```python
from build123d import *

# Parameters (mm, degrees)
F0_R     = 63.5
F0_R_2   = 44.45
F1_DEPTH = 127
F3_DEPTH = 19.05
F4_W     = 254
F4_H     = 50.8
F5_DEPTH = 152.4
F7_DEPTH = 88.9


with BuildPart() as f1:
    # F0 (on Front) → F1 (new body)
    with BuildSketch(Plane.XZ):
        Circle(F0_R)
        Circle(F0_R_2, mode=Mode.SUBTRACT)
    extrude(amount=F1_DEPTH)

    # F2 (on Front) → F3 (join)
    with BuildSketch(Plane.XZ):
        with BuildLine():
            ThreePointArc((59.227747, 22.898122), (0, -63.5), (-59.227747, 22.898122))
            Line((-59.227747, 22.898122), (-127, -152.4))
            Line((-127, -152.4), (127, -152.4))
            Line((127, -152.4), (59.227747, 22.898122))
        make_face()
    extrude(amount=F3_DEPTH)

    # F4 (on Front) → F5 (join)
    with BuildSketch(Plane.XZ):
        with Locations((0, -177.8)):
            Rectangle(F4_W, F4_H)
    extrude(amount=F5_DEPTH)

    # F6 (on face) → F7 (join)
    with BuildSketch(Plane.XZ.offset(19.05)):
        with BuildLine():
            ThreePointArc((9.525, -62.781561), (0, -63.5), (-9.525, -62.781561))
            Line((-9.525, -62.781561), (-9.525, -152.4))
            Line((-9.525, -152.4), (9.525, -152.4))
            Line((9.525, -152.4), (9.525, -62.781561))
        make_face()
    extrude(amount=F7_DEPTH)


solid = f1.part
```
Verification items for the finished model (mm, model axes). A direction names the side the tool comes from. Give positions to 0.01 mm unless a question says otherwise; leave off trailing zeros. Loops run counter-clockwise (first coordinate to the right, second up) from the corner with the lowest first, then second, coordinate; pieces in that order, holes last.
1. Go/stop test with flat-tipped pins: pin 1 Ø5 at (y, z) = (-107.5, -77) entering from -X (3 decimals); pin 2 Ø1.5 at (x, z) = (25.5, -86.5) entering from -Y; pin 3 Ø5.5 at (x, z) = (-3.5, -108.5) entering from -Y; pin 4 Ø1.5 at (x, z) = (-95, -129) entering from +Y. Record where each tip stops, or that it passes through.
2. Section check A-A, the plane y = -32. Enter the section's corners in (x, z) (3 decimals).
3. Section check D-D, the plane z = -70. Enter the section's corners in (x, y) (3 decimals), then the cut area to 3 significant figures.
4. Mould release check, pull along X, two halves, no side actions. Record for faces 5 (the flat face through (-127, -75, -178)), 6 (the flat face through (-2, -75, -203.2)), 7 (the cylindrical face through (42.397, -62.611, 13.352)): released by +X, released by -X, zero draft, split by the parting line, or undercut.
5. Section check B-B, the plane x = 0. Enter the section's corners in (y, z).
6. Set-up check for faces 1 (the flat face through (-9.525, -63, -107)), 2 (the cylindrical face through (-8.27, -62.61, 62.96)), 3 (the flat face through (9.525, -63, -108)), 4 (the flat face through (0, -107.95, -107)): record each of +Z, -Z, +X, -X, +Y, -Y from which the full face is reachable in a straight line by a thin tool's end or side.
7. Section check C-C, the plane z = 35.5. Enter the section's corners in (x, y), then the cut area to 3 significant figures.
8. Thickness scan on line 1 (Z direction, x = 0, y = -70); line 2 (Z direction, x = -31, y = -122); line 3 (X direction, y = -60, z = -1.5). Record the ranges inside material, lowest first.
Geometry says:
1. pin 1: stops at x = -9.525
1. pin 2: stops at y = -19.05
1. pin 3: stops at y = -107.95
1. pin 4: stops at y = 0
2. outline: (-127, -203.2) - (127, -203.2) - (127, -152.4) - (9.525, -152.4) - (9.525, -62.782) arc R63.5 ccw (long way) to (-9.525, -62.782) - (-9.525, -152.4) - (-127, -152.4) - close; hole circle Ø88.9 at (0, 0)
3. outline: (-95.143, -19.05) - (-9.525, -19.05) - (-9.525, -107.95) - (9.525, -107.95) - (9.525, -19.05) - (95.143, -19.05) - (95.143, 0) - (-95.143, 0) - close
3. area: 5,320 mm2
4. face 5: released by -X
4. face 6: zero draft
4. face 7: undercut
5. outline: (-152.4, -203.2) - (0, -203.2) - (0, -44.45) - (-127, -44.45) - (-127, -63.5) - (-107.95, -63.5) - (-107.95, -152.4) - (-152.4, -152.4) - close; (-127, 44.45) - (0, 44.45) - (0, 63.5) - (-127, 63.5) - close
6. face 1: -X, -Y
6. face 2: -Y
6. face 3: +X, -Y
6. face 4: +X, -X, -Y
7. outline: (-52.65, -127) - (-26.75, -127) - (-26.75, 0) - (-52.65, 0) - close; (26.75, -127) - (52.65, -127) - (52.65, 0) - (26.75, 0) - close
7. area: 6,580 mm2
8. line 1: z = -203.2 to -44.45, 44.45 to 63.5
8. line 2: z = -203.2 to -152.4, -55.42 to -31.86, 31.86 to 55.42
8. line 3: x = -63.48 to -44.42, 44.42 to 63.48
